Read the model definition and answer for the solid it produces. Units are mm, in the model's axes. Face numbers are marked on the shaded views. A direction names the side the tool comes from. Coordinates: 2 decimals unless noted, no trailing zeros. Loops run counter-clockwise (first coordinate to the right, second up) from the corner with the lowest first, then second, coordinate; pieces in that order, holes last. Notation, with made-up numbers: M 39,-18.5 L 49,-18.5 A28 cw 49,0.5 Z; hole C -6.5,-11 d8. An arc over 180 degrees is marked long. One line per item, written item: value. Start each with the question number.
1. The part is cut by section D-D (x = -3.5). Write down the section's boundary in (y, z).
2. Flat-ended cylindrical pins translate along their axes: pin 1 (5 mm diameter, centred on x = -12, y = -21.5, fed in from +Z); pin 2 (0.9 mm diameter, centred on y = 44.5, z = 1, fed in from -X); pin 3 (1.5 mm diameter, centred on x = -2, z = 1, fed in from +Y). Find the tip coordinate at first contact, or state that the pin passes through.
3. The part is cut by section C-C (z = 1.85). State how many separate pieces and enclosed holes the cut face has, then the cut area to 3 significant figures.
4. For the marked faces 1 and 2, determine the directions among +Z, -Z, +X, -X, +Y, -Y from which every point of the face is accessible in a straight line to the end or side of a thin tool.
5. Consider probe 1 along X at (y, z) = (23, 1.8); probe 2 along Y at (x, z) = (43, 1.65); probe 3 along Y at (x, z) = (-38, 2.9). Determine where each line is inside the solid, lowest interval first.
6. The part is cut by section B-B (x = -18.84). Write down the section's boundary in (y, z) (3 decimals), then the cut area to 4 significant figures.
7. The part is cut by section A-A (y = 9.5). Write down the section's boundary in (x, z), then the cut area to 3 significant figures.
8. Determine the mould class of the marked faces 3 and 4 for opening direction Y: +Y half, -Y half, draft (parallel to the pull), parting line (faces both ways), or undercut.
```python
from build123d import *

# Parameters (mm, degrees)
SKETCH1_W           = 92.97433
SKETCH1_H           = 93
BOSS_EXTRUDE1_DEPTH = 3
FILLET1_R           = 3
SKETCH4_R           = 1.6
SKETCH4_R_2         = 1.65
CUT_EXTRUDE3_DEPTH  = 3
SKETCH2_W           = 14.4
SKETCH2_H           = 2
SKETCH2_W_2         = 31.48
SKETCH2_H_2         = 4.65
SKETCH2_R           = 1.375
SKETCH2_R_2         = 0.3
CUT_EXTRUDE5_DEPTH  = 10
SKETCH2_5_R         = 0.3
CUT_EXTRUDE6_DEPTH  = 10
SKETCH2_6_R         = 1.25
CUT_EXTRUDE7_DEPTH  = 66.820259113
SKETCH2_7_R         = 1.25
CUT_EXTRUDE8_DEPTH  = 0.5
SKETCH6_R           = 6
CUT_EXTRUDE9_DEPTH  = 66.820259113
SKETCH7_R           = 0.5
SKETCH7_R_2         = 1.5
CUT_EXTRUDE10_DEPTH = 5
SKETCH7_3_W         = 15
SKETCH7_3_H         = 25
SKETCH7_3_R         = 1.5
SKETCH7_3_R_2       = 0.5
CUT_EXTRUDE11_DEPTH = 1.71


with BuildPart() as part:
    # Sketch1 → Boss-Extrude1 (new body)
    with BuildSketch(Plane.XY):
        Rectangle(SKETCH1_W, SKETCH1_H)
    extrude(amount=BOSS_EXTRUDE1_DEPTH)

    # Fillet1
    fillet1_edges = [part.edges().sort_by_distance(p)[0] for p in [
        (46.487165, -46.5, 1.5),
        (-46.487165, -46.5, 1.5),
        (-46.487165, 46.5, 1.5),
        (46.487165, 46.5, 1.5),
    ]]
    fillet(fillet1_edges, radius=FILLET1_R)

    # Sketch4 → Cut-Extrude3 (cut)
    with BuildSketch(Plane.XY.offset(3)):
        with Locations((42.777165, 39.9)):
            Circle(SKETCH4_R)
        with Locations((32.877165, 32.89)):
            Circle(SKETCH4_R_2)
    extrude(amount=-CUT_EXTRUDE3_DEPTH, mode=Mode.SUBTRACT)

    # Sketch2 → Cut-Extrude5 (cut)
    with BuildSketch(Plane.XY.offset(3)):
        with Locations((-3.98, 24.93)):
            Rectangle(SKETCH2_W, SKETCH2_H)
        with Locations((0, 44.175)):
            Rectangle(SKETCH2_W_2, SKETCH2_H_2)
        with Locations((-18.84, 21.39)):
            Circle(SKETCH2_R)
        with Locations((-21.49, 35.08)):
            Circle(SKETCH2_R_2)
        with Locations((-18.84, 44.39)):
            Circle(SKETCH2_R)
    extrude(amount=-CUT_EXTRUDE5_DEPTH, mode=Mode.SUBTRACT)

    # Sketch2_5 → Cut-Extrude6 (cut)
    with BuildSketch(Plane.XY.offset(3)):
        with Locations((-21.49, 33.81)):
            Circle(SKETCH2_5_R)
        with Locations((-21.49, 32.54)):
            Circle(SKETCH2_5_R)
        with Locations((-21.49, 31.27)):
            Circle(SKETCH2_5_R)
    extrude(amount=-CUT_EXTRUDE6_DEPTH, mode=Mode.SUBTRACT)

    # Sketch2_6 → Cut-Extrude7 (cut, through all)
    with BuildSketch(Plane.XY.offset(3)):
        with Locations((-42.988663401, 9.5)):
            Circle(SKETCH2_6_R)
        with Locations((-42.988663401, -36.5)):
            Circle(SKETCH2_6_R)
        with Locations((43.014333401, 9.5)):
            Circle(SKETCH2_6_R)
        with Locations((43.014333401, -36.5)):
            Circle(SKETCH2_6_R)
    extrude(amount=-CUT_EXTRUDE7_DEPTH, mode=Mode.SUBTRACT)

    # Sketch2_7 → Cut-Extrude8 (cut)
    with BuildSketch(Plane.XY.offset(3)):
        Polygon((-46.487165, -13.5), (-46.487165, -43.5), (46.487165, -43.5), (46.512835, 16.5), (-46.487165, 16.5), align=None)
        with Locations((-42.988663401, -36.5)):
            Circle(SKETCH2_7_R, mode=Mode.SUBTRACT)
        with Locations((-42.988663401, 9.5)):
            Circle(SKETCH2_7_R, mode=Mode.SUBTRACT)
        with Locations((43.014333401, 9.5)):
            Circle(SKETCH2_7_R, mode=Mode.SUBTRACT)
        with Locations((43.014333401, -36.5)):
            Circle(SKETCH2_7_R, mode=Mode.SUBTRACT)
    extrude(amount=-CUT_EXTRUDE8_DEPTH, mode=Mode.SUBTRACT)

    # Sketch6 → Cut-Extrude9 (cut, through all)
    with BuildSketch(Plane.XY.offset(3)):
        with Locations((31.287165, 23.5)):
            Circle(SKETCH6_R)
    extrude(amount=-CUT_EXTRUDE9_DEPTH, mode=Mode.SUBTRACT)

    # Sketch7 → Cut-Extrude10 (cut)
    with BuildSketch(Plane.XY.offset(3)):
        with Locations((-26.50049081, 42.842365948)):
            Circle(SKETCH7_R)
        with Locations((-26.50049081, 40.302365948)):
            Circle(SKETCH7_R)
        with Locations((-26.50049081, 37.762365948)):
            Circle(SKETCH7_R)
        with Locations((-26.50049081, 35.222365948)):
            Circle(SKETCH7_R)
        with Locations((-26.50049081, 32.682365948)):
            Circle(SKETCH7_R)
        with Locations((-26.50049081, 30.142365948)):
            Circle(SKETCH7_R)
        with Locations((-26.50049081, 27.602365948)):
            Circle(SKETCH7_R)
        with Locations((-26.50049081, 22.522365948)):
            Circle(SKETCH7_R)
        with Locations((-26.50049081, 19.982365948)):
            Circle(SKETCH7_R)
        with Locations((-26.50049081, 25.062365948)):
            Circle(SKETCH7_R)
        with Locations((-38.00049081, 41.662365948)):
            Circle(SKETCH7_R_2)
        with Locations((-38.00049081, 21.162365948)):
            Circle(SKETCH7_R_2)
    extrude(amount=-CUT_EXTRUDE10_DEPTH, mode=Mode.SUBTRACT)

    # Sketch7_3 → Cut-Extrude11 (cut)
    with BuildSketch(Plane.XY.offset(3)):
        with Locations((-32.50049081, 31.412365948)):
            Rectangle(SKETCH7_3_W, SKETCH7_3_H)
        with Locations((-38.00049081, 21.162365948)):
            Circle(SKETCH7_3_R, mode=Mode.SUBTRACT)
        with Locations((-38.00049081, 41.662365948)):
            Circle(SKETCH7_3_R, mode=Mode.SUBTRACT)
        with Locations((-26.50049081, 42.842365948)):
            Circle(SKETCH7_3_R_2, mode=Mode.SUBTRACT)
        with Locations((-26.50049081, 40.302365948)):
            Circle(SKETCH7_3_R_2, mode=Mode.SUBTRACT)
        with Locations((-26.50049081, 37.762365948)):
            Circle(SKETCH7_3_R_2, mode=Mode.SUBTRACT)
        with Locations((-26.50049081, 35.222365948)):
            Circle(SKETCH7_3_R_2, mode=Mode.SUBTRACT)
        with Locations((-26.50049081, 32.682365948)):
            Circle(SKETCH7_3_R_2, mode=Mode.SUBTRACT)
        with Locations((-26.50049081, 30.142365948)):
            Circle(SKETCH7_3_R_2, mode=Mode.SUBTRACT)
        with Locations((-26.50049081, 27.602365948)):
            Circle(SKETCH7_3_R_2, mode=Mode.SUBTRACT)
        with Locations((-26.50049081, 25.062365948)):
            Circle(SKETCH7_3_R_2, mode=Mode.SUBTRACT)
        with Locations((-26.50049081, 22.522365948)):
            Circle(SKETCH7_3_R_2, mode=Mode.SUBTRACT)
        with Locations((-26.50049081, 19.982365948)):
            Circle(SKETCH7_3_R_2, mode=Mode.SUBTRACT)
    extrude(amount=-CUT_EXTRUDE11_DEPTH, mode=Mode.SUBTRACT)


solid = part.part
```
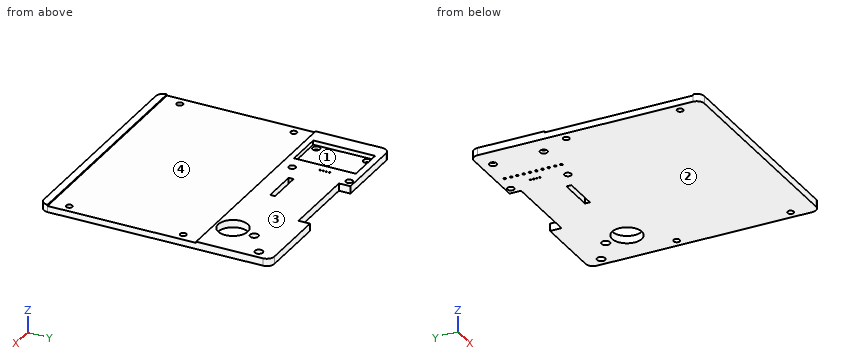
Answer block:
1. outline: M -46.5,0 L 23.93,0 L 23.93,3 L 16.5,3 L 16.5,2.5 L -43.5,2.5 L -43.5,3 L -46.5,3 Z; M 25.93,0 L 41.85,0 L 41.85,3 L 25.93,3 Z
2. pin 1: stops at z = 2.5
2. pin 2: stops at x = -46.44
2. pin 3: stops at y = 41.85
3. separate pieces: 1
3. enclosed holes: 15
3. area: 7,930 mm2
4. face 1: +Z
4. face 2: -Z, +X, -X, +Y, -Y
5. probe 1: x = -46.49 to -40, -25 to 25.31, 37.27 to 46.49
5. probe 2: y = -46.5 to -37.75, -35.25 to 8.25, 10.75 to 38.32, 41.48 to 46.5
5. probe 3: y = -46.5 to -43.5, 16.5 to 18.91, 43.91 to 46.5
6. outline: M -46.5,0 L 20.015,0 L 20.015,3 L 16.5,3 L 16.5,2.5 L -43.5,2.5 L -43.5,3 L -46.5,3 Z; M 22.765,0 L 43.015,0 L 43.015,3 L 22.765,3 Z; M 45.765,0 L 46.5,0 L 46.5,3 L 45.765,3 Z
6. area: 232.5 mm2
7. outline: M -46.49,0 L -44.24,0 L -44.24,2.5 L -46.49,2.5 Z; M -41.74,0 L 41.76,0 L 41.76,2.5 L -41.74,2.5 Z; M 44.26,0 L 46.49,0 L 46.49,2.5 L 44.26,2.5 Z
7. area: 220 mm2
8. face 3: draft
8. face 4: undercut
